from build123d import *

# Parameters (mm, degrees)
SKETCH1_R           = 75
BOSS_EXTRUDE2_DEPTH = 5
SKETCH5_W           = 35
SKETCH5_H           = 70
CUT_EXTRUDE1_DEPTH  = 107.183802908
SKETCH6_W           = 5
SKETCH6_H           = 40
BOSS_EXTRUDE3_DEPTH = 30
SKETCH7_R           = 1.6
CUT_EXTRUDE2_DEPTH  = 136.669635512
SKETCH8_W           = 40
SKETCH8_H           = 40
BOSS_EXTRUDE5_DEPTH = 12.5
SKETCH9_R           = 1.6
CUT_EXTRUDE3_DEPTH  = 111.820801297
SKETCH10_R          = 1.6
SKETCH10_R_2        = 4
CUT_EXTRUDE8_DEPTH  = 105.522724802
SKETCH13_R          = 1.5
CUT_EXTRUDE9_DEPTH  = 105.522724802
FILLET1_R           = 1
FILLET2_R           = 2


with BuildPart() as part:
    # Sketch1 → Boss-Extrude2 (new body)
    with BuildSketch(Plane(origin=(0, 0, 0), x_dir=(1, 0, 0), z_dir=(0, 1, 0))):
        with Locations(Location((0, 0, 0), (0, 0, 270))):
            Circle(SKETCH1_R)
    extrude(amount=BOSS_EXTRUDE2_DEPTH)

    # Sketch5 → Cut-Extrude1 (cut, through all)
    with BuildSketch(Plane(origin=(0, 5, 0), x_dir=(1, 0, 0), z_dir=(0, 1, 0))):
        with Locations((55, 0)):
            Rectangle(SKETCH5_W, SKETCH5_H)
        with Locations((-55, 0)):
            Rectangle(SKETCH5_W, SKETCH5_H)
    extrude(amount=-CUT_EXTRUDE1_DEPTH, mode=Mode.SUBTRACT)


with BuildPart() as cut_extrude1_piece_1:
    # of the separate pieces the step leaves, piece 1, a body of its own (cut_extrude1_pieces)
    add(part.part.solids().sort_by_distance((-66.332495807, 0, 35))[0])

    # Sketch6 → Boss-Extrude3 (add)
    with BuildSketch(Plane(origin=(0, 5, 0), x_dir=(1, 0, 0), z_dir=(0, 1, 0))):
        with Locations((-35, 0)):
            Rectangle(SKETCH6_W, SKETCH6_H)
    boss_extrude3 = extrude(amount=BOSS_EXTRUDE3_DEPTH)

    # Sketch7 → Cut-Extrude2 (cut, through all)
    with BuildSketch(Plane(origin=(-32.5, 0, 0), x_dir=(0, 0, -1), z_dir=(1, 0, 0))):
        with Locations((-8.75, 20)):
            Circle(SKETCH7_R)
        with Locations((8.75, 20)):
            Circle(SKETCH7_R)
    cut_extrude2 = extrude(amount=-CUT_EXTRUDE2_DEPTH, mode=Mode.SUBTRACT)

    # Mirror1: Boss-Extrude3, Cut-Extrude2 across plane
    add(boss_extrude3.mirror(Plane(origin=(0, 0, 0), x_dir=(0, 0, 1), z_dir=(1, 0, 0))))
    add(cut_extrude2.mirror(Plane(origin=(0, 0, 0), x_dir=(0, 0, 1), z_dir=(1, 0, 0))), mode=Mode.SUBTRACT)

    # Sketch8 → Boss-Extrude5 (add)
    with BuildSketch(Plane.XZ):
        with Locations((0, 50)):
            Rectangle(SKETCH8_W, SKETCH8_H)
    extrude(amount=BOSS_EXTRUDE5_DEPTH)

    # Sketch9 → Cut-Extrude3 (cut, through all)
    with BuildSketch(Plane.XZ.offset(12.5)):
        with Locations(Location((-15, 62, 0), (0, 0, 270))):
            Circle(SKETCH9_R)
        with Locations(Location((15, 62, 0), (0, 0, 270))):
            Circle(SKETCH9_R)
        with Locations(Location((-15, 38, 0), (0, 0, 270))):
            Circle(SKETCH9_R)
        with Locations(Location((15, 38, 0), (0, 0, 270))):
            Circle(SKETCH9_R)
    extrude(amount=-CUT_EXTRUDE3_DEPTH, mode=Mode.SUBTRACT)

    # Sketch10 → Cut-Extrude8 (cut, through all)
    with BuildSketch(Plane(origin=(0, 5, 0), x_dir=(1, 0, 0), z_dir=(0, 1, 0))):
        with Locations(Location((32.2, 27.5, 0), (0, 0, 270))):
            Circle(SKETCH10_R)
        with Locations(Location((-32.2, 27.5, 0), (0, 0, 270))):
            Circle(SKETCH10_R)
        with Locations(Location((-32.2, -27.5, 0), (0, 0, 270))):
            Circle(SKETCH10_R)
        with Locations(Location((32.2, -27.5, 0), (0, 0, 270))):
            Circle(SKETCH10_R)
        with Locations(Location((-33, 45, 0), (0, 0, 270))):
            Circle(SKETCH10_R_2)
        with Locations(Location((33, 45, 0), (0, 0, 270))):
            Circle(SKETCH10_R_2)
    extrude(amount=-CUT_EXTRUDE8_DEPTH, mode=Mode.SUBTRACT)

    # Sketch13 → Cut-Extrude9 (cut, through all)
    with BuildSketch(Plane(origin=(0, 5, 0), x_dir=(1, 0, 0), z_dir=(0, 1, 0))):
        with Locations(Location((24.25, 58, 0), (0, 0, 270))):
            Circle(SKETCH13_R)
        with Locations(Location((-24.25, 58, 0), (0, 0, 270))):
            Circle(SKETCH13_R)
        with Locations(Location((-24.25, 32, 0), (0, 0, 270))):
            Circle(SKETCH13_R)
        with Locations(Location((24.25, 32, 0), (0, 0, 270))):
            Circle(SKETCH13_R)
    extrude(amount=-CUT_EXTRUDE9_DEPTH, mode=Mode.SUBTRACT)

    # Fillet1
    fillet1_edges = [cut_extrude1_piece_1.edges().sort_by_distance(p)[0] for p in [
        (0, 5, -75),
        (0, 5, 75),
        (51.916247904, 5, 35),
        (51.916247904, 5, -35),
        (37.5, 5, -27.5),
        (-51.916247904, 5, -35),
        (-51.916247904, 5, 35),
        (-37.5, 5, 27.5),
        (-37.5, 5, -27.5),
        (37.5, 5, 27.5),
    ]]
    fillet(fillet1_edges, radius=FILLET1_R)

    # Fillet2
    fillet2_edges = [cut_extrude1_piece_1.edges().sort_by_distance(p)[0] for p in [
        (-37.5, 35, 0),
        (-32.5, 35, 0),
        (37.5, 35, 0),
        (32.5, 35, 0),
    ]]
    fillet(fillet2_edges, radius=FILLET2_R)


with BuildPart() as cut_extrude1_piece_2:
    # of the separate pieces the step leaves, piece 2, a body of its own (cut_extrude1_pieces)
    add(part.part.solids().sort_by_distance((-72.5, 0, -19.20286437))[0])


with BuildPart() as cut_extrude1_piece_3:
    # of the separate pieces the step leaves, piece 3, a body of its own (cut_extrude1_pieces)
    add(part.part.solids().sort_by_distance((72.5, 0, 19.20286437))[0])


solid = cut_extrude1_piece_1.part
Verification items for the finished model (mm, model axes). A direction names the side the tool comes from. Coordinates: 2 decimals unless noted, no trailing zeros. Order: outer loops, then holes, each group sorted by start corner. A loop starts at its lowest first (then second) coordinate and runs counter-clockwise, first axis right, second up. Notation, with made-up numbers: M -10.5,-35.75 L 2.5,-35.75 A32 cw 2.5,-2.75 Z; hole C 20.5,83.25 d5. An arc over 180 degrees is marked long. One line per item, written item: value. Start each with the question number.
Item 1: Sectioned sample at B-B on z = -15. Record the cut outline in (x, y).
Item 2: Access from +Z, -Z, +X, -X, +Y, -Y to the whole of each face (thin tool, end or side, straight path). Record for faces 4 (the flat face through (-20, -6, 50)), 5 (the flat face through (-37.5, 17, 0)), 6 (the cylindrical face through (36.966, 2.535, -45.521)), 7 (the flat face through (52, 2, -35)).
Item 3: Depth check by flat-ended pin: P1, Ø1.9, axis at x = 15, z = 38, coming from the -Y side; P2, Ø6, axis at y = -5.5, z = 40.5, coming from the -X side; P3, Ø12, axis at x = -27, y = 15.5, coming from the +Z side; P4, Ø6, axis at x = -4, y = 6.5, coming from the +Z side. Enter the tip coordinate at first touch or a pass-through.
Item 4: Sectioned sample at A-A on y = 26.5. Record the cut outline in (x, z).
Item 5: Thickness scan on probe 1 along X at (y, z) = (15, 18); probe 2 along X at (y, z) = (-8, 62); probe 3 along Y at (x, z) = (28.5, 64.5). Record the ranges inside material, lowest first.
Item 6: Mould release check, pull along Z, two halves, no side actions. Record for faces 1 (the flat face through (0, -6, 30)), 2 (the flat face through (1, 0, -18)), 3 (the cylindrical face through (16.586, -3.873, 38.208)): pulls with the +Z half, pulls with the -Z half, needs draft (parallel to the pull), parting line crosses it, or undercut.
Item 7: Sectioned sample at C-C on y = -8. Record the cut outline in (x, z), then the cut area to 3 significant figures.
Calculated:
1. outline: M -37.5,0 L 37.5,0 L 37.5,33 A2 ccw 35.5,35 L 34.5,35 A2 ccw 32.5,33 L 32.5,5 L -32.5,5 L -32.5,33 A2 ccw -34.5,35 L -35.5,35 A2 ccw -37.5,33 Z
2. face 4: +Z, -Z, -X, -Y
2. face 5: -X, +Y, -Y
2. face 6: +Y, -Y
2. face 7: +X, +Y, -Y
3. P1: through
3. P2: x = -20
3. P3: z = 20
3. P4: z = 74.96
4. outline: M -37.5,-20 L -32.5,-20 L -32.5,20 L -37.5,20 Z; M 32.5,-20 L 37.5,-20 L 37.5,20 L 32.5,20 Z
5. probe 1: -37.5 to -32.5, 32.5 to 37.5
5. probe 2: -20 to -16.6, -13.4 to 13.4, 16.6 to 20
5. probe 3: 0 to 5
6. face 1: pulls with the -Z half
6. face 2: needs draft
6. face 3: undercut
7. outline: M -20,30 L 20,30 L 20,70 L -20,70 Z; hole C -15,38 d3.2; hole C -15,62 d3.2; hole C 15,38 d3.2; hole C 15,62 d3.2
7. area: 1,570 mm^2
